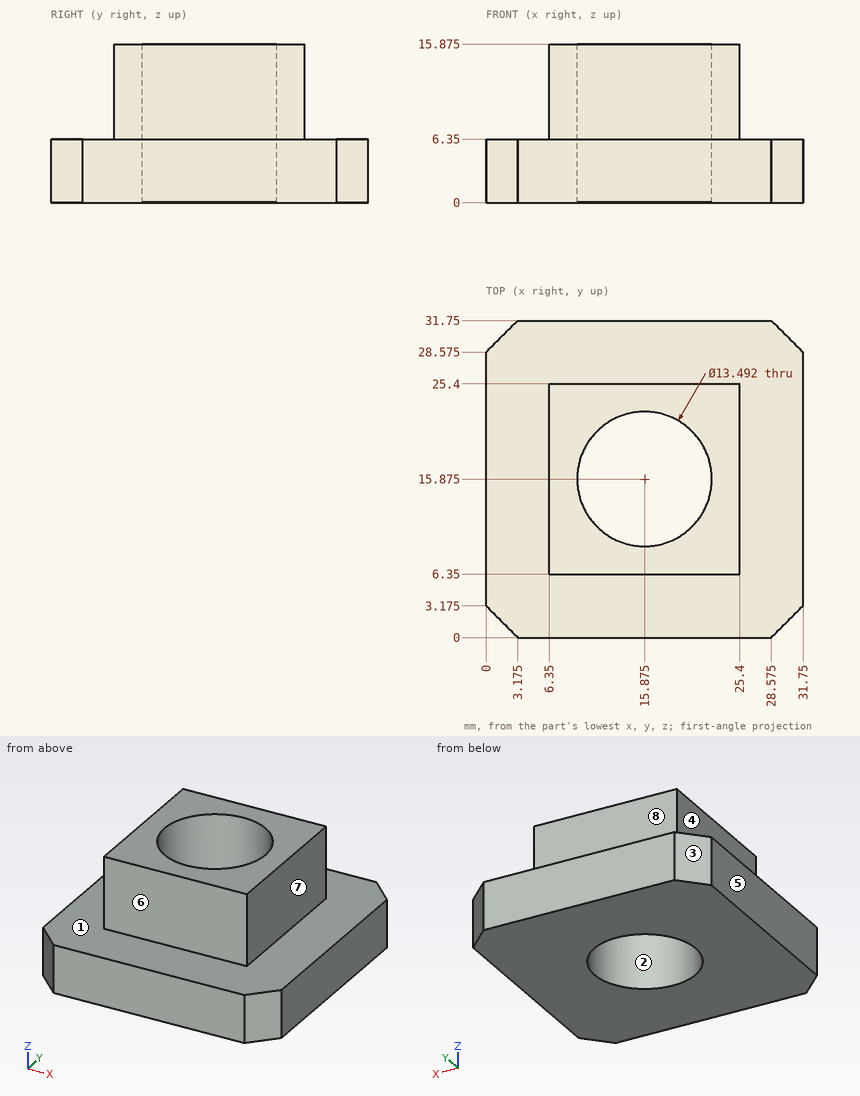
Part print with two shaded views. Sizes in mm from the minimum x, y, z corner. A direction names the side the tool comes from. Round coordinates to 2 decimals unless told otherwise and drop trailing zeros. Write each question's results on one line, items separated by ' | '.
1. Pull direction Y, two halves, no side cores. Call the marked faces 1, 2 and 3: pulls with the +Y half, pulls with the -Y half, needs draft (parallel to the pull), parting line crosses it, or undercut.
Findings below:
face 1: needs draft | face 2: undercut | face 3: pulls with the +Y half
2. Wall check: line 1 along Z through (x, y) = (28, 28); line 2 along X through (y, z) = (24, 8); line 3 along Y through (x, z) = (15.5, 6.75). Give the ranges that are in metal, low to high. Write a range as [from, to].
Findings below:
line 1: z = [0, 6.35] | line 2: x = [6.35, 25.4] | line 3: y = [6.35, 9.14], [22.61, 25.4]
3. Flat gauge pins, fed straight in: P1, Ø5, axis at x = 19, z = 10.5, coming from the -Y side; P2, Ø3, axis at x = 15.5, z = 11.5, coming from the +Y side; P3, Ø7.5, axis at y = 15.5, z = 12.5, coming from the -X side. Where does each tip first touch, or does it go through?
Findings below:
P1: stops at y = 6.35 | P2: stops at y = 25.4 | P3: stops at x = 6.35
4. 3-axis set-ups, long thin cutter, end or side, ignore diameter. For the marked faces 4, 5, 6, 7 and 8: which of +Z, -Z, +X, -X, +Y, -Y reach the whole face in a straight line?
Findings below:
face 4: +Z, -X, +Y, -Y | face 5: +Z, -Z, -X, +Y, -Y | face 6: +Z, +X, -X, -Y | face 7: +Z, +X, +Y, -Y | face 8: +Z, +X, -X, +Y
